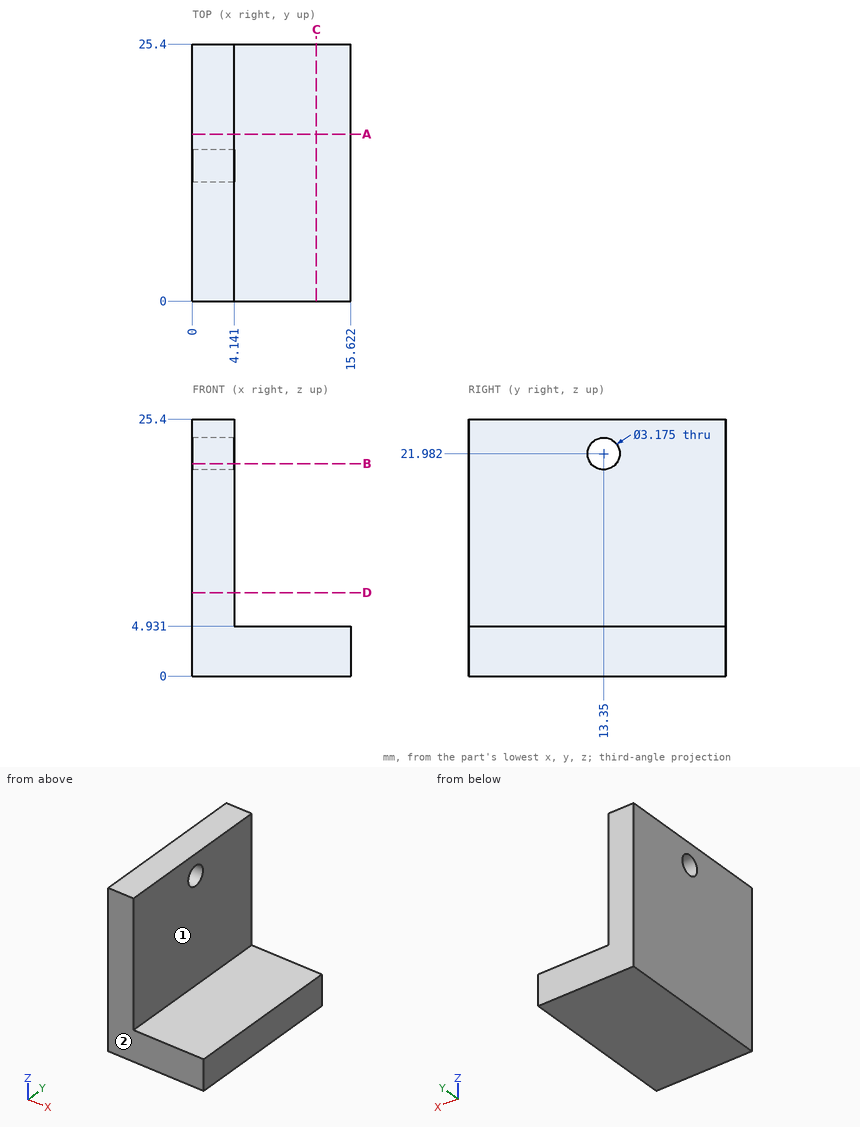
Input: dimensioned drawing with shaded views. Units: mm. Origin: part minimum x, y, z. A direction names the side the tool comes from. Round coordinates to 2 decimals unless told otherwise and drop trailing zeros. Order: outer loops, then holes, each group sorted by start corner. A loop starts at its lowest first (then second) coordinate and runs counter-clockwise, first axis right, second up. Notation, with made-up numbers: (-4, 32.5) -> (31, 32.5) arc R27 ccw to (31, 60.5) -> close; hole circle Ø4 at (89.5, 81.5). An arc over 180 degrees is marked (long way). Put each result on its own line as item: value. Start each with the question number.
Q1. First-contact query: pin 1 (3 mm diameter, centred on y = 13.35, z = 21.98, fed in from -X); pin 2 (9 mm diameter, centred on x = 9.5, y = 11.5, fed in from +Z); pin 3 (2 mm diameter, centred on y = 13.5, z = 12.5, fed in from +X). Flat tips, straight axial feed; report the tip coordinate or a pass-through.
Q2. Line query: probe 1 along X at (y, z) = (20.75, 20); probe 2 along Z at (x, y) = (13.5, 6); probe 3 along Z at (x, y) = (3.75, 14) (1 decimal). Output: solid intervals per line, ascending.
Q3. Section B-B on z = 21. Return the cut outline in (x, y).
Q4. Section C-C on x = 12.25. Return the cut outline in (y, z).
Q5. Section A-A on y = 16.5. Return the cut outline in (x, z), and give its area (3 significant figures).
Q6. Section D-D on z = 8.25. Return the cut outline in (x, y).
Q7. Reachability of the marked faces 1 and 2 from +Z, -Z, +X, -X, +Y, -Y: full face, straight path, thin tool, end or side. Return the list, or none.
Ans:
1. pin 1: passes through
1. pin 2: stops at z = 4.93
1. pin 3: stops at x = 4.14
2. probe 1: x = 0 to 4.14
2. probe 2: z = 0 to 4.93
2. probe 3: z = 0 to 20.5, 23.4 to 25.4
3. outline: (0, 0) -> (4.14, 0) -> (4.14, 12.1) -> (0, 12.1) -> close; (0, 14.6) -> (4.14, 14.6) -> (4.14, 25.4) -> (0, 25.4) -> close
4. outline: (0, 0) -> (25.4, 0) -> (25.4, 4.93) -> (0, 4.93) -> close
5. outline: (0, 0) -> (15.62, 0) -> (15.62, 4.93) -> (4.14, 4.93) -> (4.14, 25.4) -> (0, 25.4) -> close
5. area: 162 mm2
6. outline: (0, 0) -> (4.14, 0) -> (4.14, 25.4) -> (0, 25.4) -> close
7. face 1: +Z, +X, +Y, -Y
7. face 2: +Z, -Z, +X, -X, -Y
